Work out the finished part from the listing and answer in its coordinate system (mm). A direction names the side the tool comes from. Coordinates: 2 decimals unless noted, no trailing zeros. Write each loop counter-clockwise with the first axis right and the second up, starting at its lowest first coordinate (ties: lowest second). Pieces come first, ordered by that corner, then holes. Notation, with made-up numbers: (10.25, -31.75) - (14.25, -31.75) arc R16 ccw to (14.25, -8.75) - close; hole circle Ø3 at (-21, 64.5). An arc over 180 degrees is marked (long way). Use one line per item in the form item = value. Start each with the question number.
Item 1: Determine the mould class of faces 3 (the flat face through (-4, 0, 6.35)), 4 (the cylindrical face through (-9.442, 0.001, 3.131)), 5 (the cylindrical face through (0.688, 8.013, 3.131)), 6 (the flat face through (-3.572, -6, 3)) for opening direction Y: released by +Y, released by -Y, zero draft, split by the parting line, or undercut.
Item 2: A cutting plane is placed at D-D (x = -2.75). Write down the section's boundary in (y, z).
Item 3: A cutting plane is placed at C-C (z = 3). Give the number of separate pieces and of enclosed holes in the cut face, then the cut area to 3 significant figures.
Item 4: For faces 1 (the flat face through (-4, 0, 0)), 2 (the cylindrical face through (0.079, -13.096, 3.131)), determine the directions among +Z, -Z, +X, -X, +Y, -Y from which every point of the face is accessible in a straight line to the end or side of a thin tool.
Item 5: A cutting plane is placed at A-A (y = -6.5). Write down the section's boundary in (x, z) (3 decimals).
Item 6: A cutting plane is placed at B-B (x = 0). Write down the section's boundary in (y, z).
Item 7: Consider probe 1 along Y at (x, z) = (0, 2.75); probe 2 along Y at (x, z) = (0.75, 4); probe 3 along X at (y, z) = (-8, 2). Determine where each line is inside the solid, lowest interval first.
Item 8: Given pin 1 (2 mm diameter, centred on x = -4.5, z = 5.5, fed in from -Y); pin 2 (1 mm diameter, centred on x = -0.5, y = 12, fed in from +Z), each flat-ended and moving along its own axis, determine where each tip first touches the part or whether it passes through.
from build123d import *

# Parameters (mm, degrees)
BASE_FLANGE1_DEPTH              = 6.35
F_1_4_0_25_DIAMETER_HOLE1_D     = 6.35
F_9_32_0_28125_DIAMETER_HOLE1_D = 7.14375
CUT_EXTRUDE1_REACH              = 22.88
CUT_EXTRUDE2_DEPTH              = 21.88030247
FILLET1_R                       = 6.35


# Sheet-metal steps are written as plain solids
with BuildPart() as part:
    # Sketch1 → Base-Flange1 (new body)
    with BuildSketch(Plane.XY):
        with BuildLine():
            Line((9.525, 7.9375), (9.525, -7.9375))
            ThreePointArc((9.525, -7.9375), (0, -17.4625), (-9.525, -7.9375))
            Line((-9.525, -7.9375), (-9.525, 7.9375))
            ThreePointArc((-9.525, 7.9375), (0, 17.4625), (9.525, 7.9375))
        make_face()
    extrude(amount=BASE_FLANGE1_DEPTH)

    # 1/4 (0.25) Diameter Hole1 (through all)
    with Locations(Plane.XY.offset(6.35)):
        with Locations((0, 11.1125)):
            Hole(F_1_4_0_25_DIAMETER_HOLE1_D / 2)

    # 9/32 (0.28125) Diameter Hole1 (through all)
    with Locations(Plane.XY.offset(6.35)):
        with Locations((0, -9.525)):
            Hole(F_9_32_0_28125_DIAMETER_HOLE1_D / 2)

    # Sketch6 → Cut-Extrude1 (cut, up to next)
    with BuildSketch(Plane.XY.offset(6.35), mode=Mode.PRIVATE) as cut_extrude1_sk1:
        with BuildLine():
            Line((-3.571875, -9.525), (-3.571875, -1.5875))
            ThreePointArc((-3.571875, -1.5875), (0, 1.984375), (3.571875, -1.5875))
            Line((3.571875, -1.5875), (3.571875, -9.525))
            ThreePointArc((3.571875, -9.525), (0, -13.096875), (-3.571875, -9.525))
        make_face()
    cut_extrude1_tool1 = extrude(cut_extrude1_sk1.sketch, amount=-CUT_EXTRUDE1_REACH, mode=Mode.PRIVATE) & part.part
    add(cut_extrude1_tool1.solids().sort_by_distance((0, -5.55625, 6.35))[0], mode=Mode.SUBTRACT)

    # Sketch7 → Cut-Extrude2 (cut, through all)
    with BuildSketch(Plane.XY.offset(6.35)):
        with BuildLine():
            Line((-4.336848919, 16.417910748), (-9.525, 0))
            Line((-9.525, 0), (-5.27553043, 12.856258225))
            ThreePointArc((-5.27553043, 12.856258225), (-3.89412581, 15.075793862), (-1.650615296, 16.417910748))
            Line((-1.650615296, 16.417910748), (-4.336848919, 16.417910748))
        make_face()
        with BuildLine():
            ThreePointArc((1.650615296, 16.417910748), (3.89412581, 15.075793862), (5.27553043, 12.856258225))
            Line((5.27553043, 12.856258225), (9.525, 0))
            Line((9.525, 0), (4.336848919, 16.417910748))
            Line((4.336848919, 16.417910748), (1.650615296, 16.417910748))
        make_face()
        with BuildLine():
            ThreePointArc((9.525, 7.9375), (8.125088029, 12.908271522), (4.336848919, 16.417910748))
            Line((4.336848919, 16.417910748), (9.525, 0))
            Line((9.525, 0), (9.525, 7.9375))
        make_face()
        with BuildLine():
            Line((-9.525, 7.9375), (-9.525, 0))
            Line((-9.525, 0), (-4.336848919, 16.417910748))
            ThreePointArc((-4.336848919, 16.417910748), (-8.125088029, 12.908271522), (-9.525, 7.9375))
        make_face()
        with BuildLine():
            ThreePointArc((-1e-09, 17.4625), (-2.230438592, 17.197671094), (-4.336848919, 16.417910748))
            Line((-4.336848919, 16.417910748), (-1.650615296, 16.417910748))
            ThreePointArc((-1.650615296, 16.417910748), (0, 16.66875), (1.650615296, 16.417910748))
            Line((1.650615296, 16.417910748), (4.336848919, 16.417910748))
            ThreePointArc((4.336848919, 16.417910748), (2.230438592, 17.197671094), (-1e-09, 17.4625))
        make_face()
    extrude(amount=-CUT_EXTRUDE2_DEPTH, mode=Mode.SUBTRACT)

    # Fillet1
    fillet1_edges = [part.edges().sort_by_distance(p)[0] for p in [
        (9.525, 0, 3.175),
        (-9.525, 0, 3.175),
    ]]
    fillet(fillet1_edges, radius=FILLET1_R)


solid = part.part
Answer:
q1.face_3 = zero draft
q1.face_4 = released by +Y
q1.face_5 = undercut
q1.face_6 = undercut
q2.outline = (-17.06, 0) - (-11.8, 0) - (-11.8, 6.35) - (-17.06, 6.35) - close; (0.69, 0) - (9.53, 0) - (9.53, 6.35) - (0.69, 6.35) - close; (12.7, 0) - (15.94, 0) - (15.94, 6.35) - (12.7, 6.35) - close
q3.separate_pieces = 1
q3.enclosed_holes = 2
q3.area = 385 mm²
q4.face_1 = -Z, +X, -X, +Y, -Y
q4.face_2 = +Z, -Z
q5.outline = (-9.525, 0) - (-3.572, 0) - (-3.572, 6.35) - (-9.525, 6.35) - close; (3.572, 0) - (9.525, 0) - (9.525, 6.35) - (3.572, 6.35) - close
q6.outline = (-17.46, 0) - (-13.1, 0) - (-13.1, 6.35) - (-17.46, 6.35) - close; (1.98, 0) - (7.94, 0) - (7.94, 6.35) - (1.98, 6.35) - close; (14.29, 0) - (16.67, 0) - (16.67, 6.35) - (14.29, 6.35) - close
q7.probe_1 = -17.46 to -13.1, 1.98 to 7.94, 14.29 to 16.67
q7.probe_2 = -17.43 to -13.02, 1.9 to 8.03, 14.2 to 16.62
q7.probe_3 = -9.52 to -3.57, 3.57 to 9.52
q8.pin_1 = -16.8
q8.pin_2 = through
